For this review, take the finished solid that the model builds, in its own axes (mm). Face numbers are marked on the shaded views. A direction names the side the tool comes from. Give positions to 0.01 mm unless a question says otherwise; leave off trailing zeros. Order: outer loops, then holes, each group sorted by start corner. A loop starts at its lowest first (then second) coordinate and runs counter-clockwise, first axis right, second up. Notation, with made-up numbers: (-11.75, -7) -> (13.25, -7) arc R34 cw to (13.25, 27) -> close; hole circle Ø8 at (55, 86). An arc over 180 degrees is marked (long way). Use CSV: the item, a comma, the result in double quotes. Start each with the question number.
Autodesk Fusion 360 part; units mm, degrees
sketch "Base profile and screw holes" plane through (0, 0, 0) normal (0, 0, 1) x (1, 0, 0)
  line L0 (15, 15) -> (-15, 15)
  line L1 (-15, 15) -> (-15, -17)
  line L2 (-15, -17) -> (15, -17)
  line L3 (15, -17) -> (15, 15)
  circle A0 centre (-11, -11) radius 1.25
  circle A1 centre (9, -11) radius 1.25
  circle A2 centre (-11, 9) radius 1.25
  circle A3 centre (9, 9) radius 1.25
  dimension "d1" = 30
  dimension "d5" = 4
  dimension "d8" = 20
  dimension "d9" = 2.5
  dimension "d10" = 20
  dimension "d40" = 11
  dimension "d41" = 6
  dimension "d42" = 6
extrude "Extrude1" add sketch "Base profile and screw holes" along normal blind 10 makes body 1
ref_plane "WorkPlane1" through (0, 0, -30) normal (0, 0, 1) x (1, 0, 0)
sketch "Original holder" plane through (0, 0, -30) normal (0, 0, 1) x (1, 0, 0)
  circle A0 centre (-31, 0) radius 12.75
  circle A1 centre (-11, -11) radius 1.25
  line L0 (-14.1024, 16) -> (-47.8976, 16)
  line L1 (-47.8976, 16) -> (-47.8976, -16)
  line L2 (-47.8976, -16) -> (-14.1024, -16)
  line L3 (-14.1024, -16) -> (-14.1024, 16)
  line L4 (-14.1024, 16) -> (-47.8976, -16) construction
  line L5 (-47.8976, 16) -> (-14.1024, -16) construction
  line L6 (-15, 15) -> (-15, -17)
  point P0 (-31, 0)
  dimension "d16" = 25.5
  dimension "d17" = 20
extrude "Extrude2" add sketch "Original holder" against normal blind 5 separate body contours L0 L1 L2 L3 makes body 2
sketch "Nikon 10x objective" plane through (0, 0, 0) normal (0, 1, 0) x (1, 0, 0)
  line L0 (-43.4233, 29.7385) -> (-30.9233, 29.7385)
  line L1 (-30.9233, 29.7385) -> (-30.9233, 34.7385)
  line L2 (-30.9233, 34.7385) -> (-43.4233, 34.7385)
  line L3 (-43.4233, 34.7385) -> (-43.4233, 29.7385)
  line L4 (-30.9233, 29.7385) -> (-44.9233, 29.7385)
  line L5 (-44.9233, 29.7385) -> (-44.9233, 24.7385)
  line L6 (-44.9233, 24.7385) -> (-30.9233, 24.7385)
  line L7 (-30.9233, 24.7385) -> (-30.9233, 29.7385)
  line L8 (-44.9233, 24.7385) -> (-42.9233, 22.7376)
  line L9 (-44.9233, 24.7385) -> (-39.0718, 24.7385) construction
  line L10 (-30.9233, 24.7385) -> (-42.9233, 24.7385)
  line L11 (-42.9233, 24.7385) -> (-42.9233, -13.2615)
  line L12 (-42.9233, -13.2615) -> (-30.9233, -13.2615)
  line L13 (-30.9233, -13.2615) -> (-30.9233, 24.7385)
  line L14 (-30.9233, -13.2615) -> (-40.1733, -13.2615)
  line L15 (-40.1733, -13.2615) -> (-40.1733, -16.7692)
  line L16 (-30.9233, -17.6525) -> (-30.9233, -13.2615)
  line L17 (-40.1733, -16.7692) -> (-34.1733, -27.1615)
  line L18 (-30.9233, -17.6525) -> (-30.9233, -27.1615)
  line L19 (-34.1733, -27.1615) -> (-30.9233, -27.1615)
  line L20 (-42.9233, -10.9477) -> (-41.5874, -13.2615)
  line L21 (-42.9233, -10.9477) -> (-41.0507, -10.9477) construction
  dimension "d20" = 12.5
  dimension "d21" = 5
  dimension "d22" = 14
  dimension "d23" = 5
  dimension "d26" = 12
  dimension "d29" = 9.25
  dimension "d31" = 3.25
  dimension "d33" = 43
  dimension "d34" = 60
  dimension "d35" = 13.9
  dimension "d36" = 60
revolve "Revolve1" add sketch "Nikon 10x objective" angle 360 about axis through (-30.9233, 0, 13.2615) along (0, 0, -1) separate body contours L0 L1 L2 L3 L4 | L0 L4 L5 L6 L7 L10 | L6 L10 L11 L12 L13 L14 L20 | L6 L8 L11 | L12 L14 L15 L16 L17 L18 L19 makes body 3
sketch "Main body of holder" plane through (0, 0, 0) normal (0, 0, 1) x (1, 0, 0)
  circle A0 centre (-31, -1) radius 12
  line L0 (-11, 9) -> (-11, -11) construction
  line L1 (-15, 15) -> (-59, 15)
  line L2 (-59, 15) -> (-59, -17)
  line L3 (-59, -17) -> (-15, -17)
  line L4 (-15, -17) -> (-15, 15)
  line L5 (-59, -9) -> (-39.9443, -9)
  line L6 (-59, 0) -> (-42.9583, 0)
  point P0 (-11, -11)
  point P1 (-11, 9)
  point P2 (-11, -1)
  point P3 (-15, 15)
  point P4 (-15, -17)
  dimension "d38" = 24
  dimension "d39" = 20
  dimension "d43" = 15
  dimension "d44" = 8
  dimension "d45" = 44
extrude "Extrude3" add sketch "Main body of holder" along normal up to surface (10 mm away) contours A0 L1 L2 L3 L4 L5 L6 bodies 1
sketch "Hole for bolt that goes into heat-set insert" plane through (0, -17, 0) normal (0, -1, 0) x (1, 0, 0)
  line L0 (-59, 0) -> (15, 0)
  line L1 (15, 0) -> (15, 10)
  line L2 (15, 10) -> (-59, 10)
  line L3 (-59, 10) -> (-59, 0)
  circle A0 centre (-51.5415, 5) radius 1.75
  point P0 (-59, 5)
  dimension "d48" = 3.5
extrude "Extrude4" cut sketch "Hole for bolt that goes into heat-set insert" against normal up to surface (8 mm away) contours A0 bodies 1
chamfer "Chamfer1" distance 2 angle 45 1 edges at (-39.9443, -9, 5) on bodies 1
sketch "Hole for heat-set insert" plane through (0, 15, 0) normal (0, 1, 0) x (-1, 0, 0)
  line L0 (-15, 0) -> (59, 0)
  line L1 (59, 0) -> (59, 10)
  line L2 (59, 10) -> (-15, 10)
  line L3 (-15, 10) -> (-15, 0)
  circle A0 centre (51.5415, 5) radius 2.6
  circle A1 centre (51.5415, 5) radius 1.75
  dimension "d52" = 5.2
extrude "Extrude5" cut sketch "Hole for heat-set insert" against normal up to surface (15 mm away) contours A0 | A1 bodies 1
fillet "Fillet3" radius 2 7 edges at (-59, 15, 5) (-59, 0, 5) (-59, -9, 5) (-59, -17, 5) (-42.9583, 0, 5) (15, -17, 5) (15, 15, 5) on bodies 1
chamfer "Chamfer2" distance 0.2 angle 45 34 edges at (-22, 15, 10) (14.4142, 14.4142, 10) (15, -1, 10) (14.4142, -16.4142, 10) (-22, -17, 10) (-58.4142, -16.4142, 10) (-59, -13, 10) (-58.4142, -9.5858, 10) (-49.4721, -9, 10) (-19.6882, 3.0054, 10) (-43.4212, 0.4416, 10) (-50.8374, 0, 10) (-58.4142, 0.5858, 10) (-59, 7.5, 10) (-58.4142, 14.4142, 10) (-22, 15, 0) (14.4142, 14.4142, 0) (15, -1, 0) (14.4142, -16.4142, 0) (-22, -17, 0) (-58.4142, -16.4142, 0) (-59, -13, 0) (-58.4142, -9.5858, 0) (-49.4721, -9, 0) (-19.6882, 3.0054, 0) (-43.4212, 0.4416, 0) (-50.8374, 0, 0) (-58.4142, 0.5858, 0) (-59, 7.5, 0) (-58.4142, 14.4142, 0) (-12.1654, -10.548, 0) (-12.1654, 9.452, 0) (7.8346, 9.452, 0) (7.8346, -10.548, 0) on bodies 1
chamfer "Chamfer2" distance 0.2 angle 45 2 edges at (-40.2178, -9.6872, 0) (-40.2178, -9.6872, 10) on bodies 1
sketch "Counterbore for bolts that attach to microscope stage" plane through (0, 0, 10) normal (0, 0, 1) x (-1, 0, 0)
  circle A0 centre (11, -9) radius 2.5
  circle A1 centre (-9, -9) radius 2.5
  circle A2 centre (11, 11) radius 2.5
  circle A3 centre (-9, 11) radius 2.5
  point P0 (11, -9)
  point P1 (-9, -9)
  point P2 (-9, 11)
  point P3 (11, 11)
  dimension "d62" = 5
extrude "Extrude6" cut sketch "Counterbore for bolts that attach to microscope stage" against normal blind 2.2 bodies 1
sketch "Counterbore for bolt that goes into the heat-set insert" plane through (0, 15, 0) normal (0, -1, 0) x (1, 0, 0)
  circle A0 centre (-51.5415, 5) radius 3.3
  point P0 (-51.5415, 5)
  dimension "d65" = 6.6
extrude "Extrude8" cut sketch "Counterbore for bolt that goes into the heat-set insert" along normal blind 7 bodies 1
hidden bodies 2 3
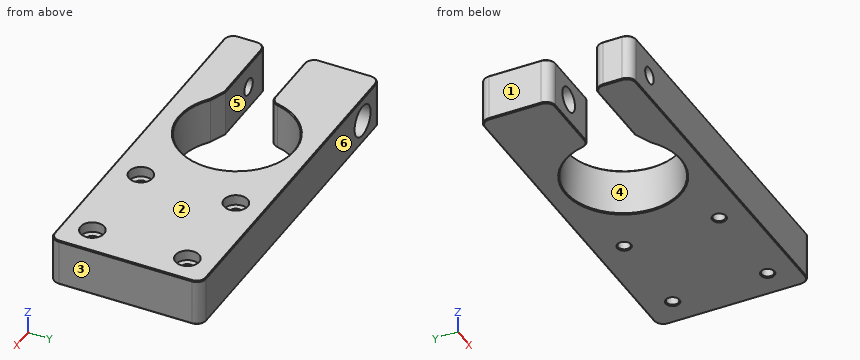
1. Draft analysis for pull direction X (two halves, no side actions). For the marked faces 1, 2, 3 and 4, state which applies: +X half, -X half, draft (parallel to the pull), parting line (faces both ways), or undercut.
2. Consider section B-B (x = -31). State the section outline as (y, z) points, plus the area to 3 significant figures.
3. Consider section D-D (y = 9). State how many separate pieces and enclosed holes the cut face has, plus the area to 3 significant figures.
4. To check wall thickness, follow L1, parallel to Y at x = 9, z = 4.5; L2, parallel to X at y = -11, z = 8.8; L3, parallel to X at y = -11, z = 6.25. State the ranges of each line that lie inside material, in increasing order. Write a range as [from, to].
5. Consider section C-C (y = -1). State the section outline as (x, z) points.
6. Clearance check with flat-ended pins moving along their axes: P1, Ø2.5, axis at x = 9.5, y = -11, coming from the +Z side; P2, Ø4, axis at y = -4, z = 4.5, coming from the -X side. State where each tip first meets the part, or that it passes through.
7. For the marked faces 5 and 6, list the 3-axis set-ups (+Z, -Z, +X, -X, +Y, -Y) from which the entire face can be reached by the end or side of a thin tool; tool diameter is ignored.
8. Consider section A-A (x = 9). State the section outline as (y, z) points, plus the area to 3 significant figures.
Answer list:
1,face 1,"-X half"
1,face 2,"draft"
1,face 3,"+X half"
1,face 4,"undercut"
2,outline,"(-17, 0.2) -> (-16.8, 0) -> (-13.2, 0) -> (-13, 0.2) -> (-13, 9.8) -> (-13.2, 10) -> (-16.8, 10) -> (-17, 9.8) -> close; (11, 0.2) -> (11.2, 0) -> (14.8, 0) -> (15, 0.2) -> (15, 9.8) -> (14.8, 10) -> (11.2, 10) -> (11, 9.8) -> close"
2,area,"79.8 mm2"
3,separate pieces,"4"
3,enclosed holes,"1"
3,area,"512 mm2"
4,L1,"[-17, -12.25], [-9.75, 7.75], [10.25, 15]"
4,L2,"[-59, -37.63], [-24.37, -13.5], [-8.5, 6.5], [11.5, 15]"
4,L3,"[-59, -52.77], [-50.32, -37.63], [-24.37, -12.25], [-9.75, 7.75], [10.25, 15]"
5,outline,"(-19, 0.2) -> (-18.8, 0) -> (14.8, 0) -> (15, 0.2) -> (15, 9.8) -> (14.8, 10) -> (-18.8, 10) -> (-19, 9.8) -> close"
6,P1,"z = 7.8"
6,P2,"x = -20.09"
7,face 5,"+Z, -Z, -X"
7,face 6,"+Z, -Z, +X, -X, +Y"
8,outline,"(-17, 0.2) -> (-16.8, 0) -> (-12.45, 0) -> (-12.25, 0.2) -> (-12.25, 7.8) -> (-13.5, 7.8) -> (-13.5, 10) -> (-16.8, 10) -> (-17, 9.8) -> close; (-9.75, 0.2) -> (-9.55, 0) -> (7.55, 0) -> (7.75, 0.2) -> (7.75, 7.8) -> (6.5, 7.8) -> (6.5, 10) -> (-8.5, 10) -> (-8.5, 7.8) -> (-9.75, 7.8) -> close; (10.25, 0.2) -> (10.45, 0) -> (14.8, 0) -> (15, 0.2) -> (15, 9.8) -> (14.8, 10) -> (11.5, 10) -> (11.5, 7.8) -> (10.25, 7.8) -> close"
8,area,"259 mm2"
